from build123d import *

# Parameters (mm, degrees)
EXTRUDE_THIN1_DEPTH = 736.6
CUT_EXTRUDE2_DEPTH  = 738.475341961
SKETCH5_R           = 2.0193
CUT_EXTRUDE3_DEPTH  = 738.475341961


with BuildPart() as part:
    # Sketch1 → Extrude-Thin1 (new body)
    with BuildSketch(Plane.XY):
        with BuildLine():
            Line((-10.16, 25.4), (10.16, 25.4))
            ThreePointArc((10.16, 25.4), (11.956051224, 24.656051224), (12.7, 22.86))
            Line((12.7, 22.86), (12.7, -22.86))
            ThreePointArc((12.7, -22.86), (11.956051224, -24.656051224), (10.16, -25.4))
            Line((10.16, -25.4), (-10.16, -25.4))
            ThreePointArc((-10.16, -25.4), (-11.956051224, -24.656051224), (-12.7, -22.86))
            Line((-12.7, -22.86), (-12.7, 22.86))
            ThreePointArc((-12.7, 22.86), (-11.956051224, 24.656051224), (-10.16, 25.4))
        make_face()
        with BuildLine():
            Line((-10.16, 23.749), (10.16, 23.749))
            ThreePointArc((10.16, 23.749), (10.788617928, 23.488617928), (11.049, 22.86))
            Line((11.049, 22.86), (11.049, -22.86))
            ThreePointArc((11.049, -22.86), (10.788617928, -23.488617928), (10.16, -23.749))
            Line((10.16, -23.749), (-10.16, -23.749))
            ThreePointArc((-10.16, -23.749), (-10.788617928, -23.488617928), (-11.049, -22.86))
            Line((-11.049, -22.86), (-11.049, 22.86))
            ThreePointArc((-11.049, 22.86), (-10.788617928, 23.488617928), (-10.16, 23.749))
        make_face(mode=Mode.SUBTRACT)
    extrude(amount=EXTRUDE_THIN1_DEPTH)

    # Sketch3 → Cut-Extrude2 (cut, through all)
    with BuildSketch(Plane.ZY.offset(12.7)):
        with BuildLine():
            Line((558.8, -6.35), (419.1, -6.35))
            ThreePointArc((419.1, -6.35), (412.75, 0), (419.1, 6.35))
            Line((419.1, 6.35), (558.8, 6.35))
            ThreePointArc((558.8, 6.35), (565.15, 0), (558.8, -6.35))
        make_face()
    extrude(amount=-CUT_EXTRUDE2_DEPTH, mode=Mode.SUBTRACT)

    # Sketch5 → Cut-Extrude3 (cut, through all)
    with BuildSketch(Plane(origin=(12.7, 0, 0), x_dir=(0, 0, -1), z_dir=(1, 0, 0))):
        with Locations((-393.7, 17.399)):
            Circle(SKETCH5_R)
        with Locations((-393.7, -17.399)):
            Circle(SKETCH5_R)
        with Locations((-488.95, 17.399)):
            Circle(SKETCH5_R)
        with Locations((-488.95, -17.399)):
            Circle(SKETCH5_R)
        with Locations((-584.2, -17.399)):
            Circle(SKETCH5_R)
        with Locations((-584.2, 17.399)):
            Circle(SKETCH5_R)
    extrude(amount=-CUT_EXTRUDE3_DEPTH, mode=Mode.SUBTRACT)


solid = part.part
Work out the finished part from the listing and answer in its coordinate system (mm). A direction names the side the tool comes from. Round coordinates to 2 decimals unless told otherwise and drop trailing zeros. Write each loop counter-clockwise with the first axis right and the second up, starting at its lowest first coordinate (ties: lowest second). Pieces come first, ordered by that corner, then holes.
1) A tool of negligible diameter and unlimited length cuts with its end or side. For faces 4 (the flat face through (-11.049, 0, 363)), 5 (the flat face through (-11.2, 0.1, 0)), from which of +Z, -Z, +X, -X, +Y, -Y can it reach the whole face along a straight path? Write none if from no direction.
2) A cutting plane is placed at B-B (y = 0). Give the vertices of the cut face in (x, z).
3) The mould has two halves that part along Y. Classify faces 1 (the flat face through (-12.7, 0, 363)), 2 (the flat face through (0, 25.4, 363)), 3 (the flat face through (11.049, 0, 363)): pulls with the +Y half, pulls with the -Y half, needs draft (parallel to the pull), parting line crosses it, or undercut.
4) A cutting plane is placed at C-C (z = 94.5). Give the vertices of the cut face in (x, y), plus the area to 3 significant figures.
5) Given pin 1 Ø0.5 at (x, z) = (12, 482) entering from +Y; pin 2 Ø0.8 at (x, z) = (12, 503) entering from -Y; pin 3 Ø0.5 at (x, z) = (-12, 494) entering from -Y, each flat-ended and moving along its own axis, determine where each tip first touches the part or whether it passes through.
6) A cutting plane is placed at A-A (x = -1.75). Give the vertices of the cut face in (y, z), plus the area to 3 significant figures.
7) Straight lines are drawn through the part: line 1 (Y direction, x = -6, z = 604); line 2 (X direction, y = 22.5, z = 213.5); line 3 (Y direction, x = -12.35, z = 393.7). For each, find the intervals that lie inside material, in ascending order.
Completed:
1. face 4: +Z, -Z
1. face 5: -Z, +X, -X, +Y, -Y
2. outline: (-12.7, 0) - (-11.05, 0) - (-11.05, 412.75) - (-12.7, 412.75) - close; (-12.7, 565.15) - (-11.05, 565.15) - (-11.05, 736.6) - (-12.7, 736.6) - close; (11.05, 0) - (12.7, 0) - (12.7, 412.75) - (11.05, 412.75) - close; (11.05, 565.15) - (12.7, 565.15) - (12.7, 736.6) - (11.05, 736.6) - close
3. face 1: needs draft
3. face 2: pulls with the +Y half
3. face 3: undercut
4. outline: (-12.7, -22.86) arc R2.54 ccw to (-10.16, -25.4) - (10.16, -25.4) arc R2.54 ccw to (12.7, -22.86) - (12.7, 22.86) arc R2.54 ccw to (10.16, 25.4) - (-10.16, 25.4) arc R2.54 ccw to (-12.7, 22.86) - close; hole (-11.05, -22.86) arc R0.89 ccw to (-10.16, -23.75) - (10.16, -23.75) arc R0.89 ccw to (11.05, -22.86) - (11.05, 22.86) arc R0.89 ccw to (10.16, 23.75) - (-10.16, 23.75) arc R0.89 ccw to (-11.05, 22.86) - close
4. area: 236 mm2
5. pin 1: stops at y = 24.84
5. pin 2: stops at y = -24.95
5. pin 3: stops at y = -24.84
6. outline: (-25.4, 0) - (-23.75, 0) - (-23.75, 736.6) - (-25.4, 736.6) - close; (23.75, 0) - (25.4, 0) - (25.4, 736.6) - (23.75, 736.6) - close
6. area: 2,430 mm2
7. line 1: y = -25.4 to -23.75, 23.75 to 25.4
7. line 2: x = -12.7 to -11.05, 11.05 to 12.7
7. line 3: y = -24.15 to -19.42, -15.38 to 15.38, 19.42 to 24.15
